Answer from the drawing. Dimensions are ordinates in mm from the lowest x, y and z of the part. Give positions to 0.01 mm unless a question says otherwise; leave off trailing zeros. Write each loop counter-clockwise with the first axis right and the second up, starting at its lowest first coordinate (ties: lowest second). Pieces come first, ordered by that corner, then holes. Notation, with made-up numbers: (50.25, -26) - (70.25, -26) arc R15 cw to (70.25, -3) - close; hole circle Ø2 at (-14.75, 9). An arc over 180 degrees is marked (long way). Write item = value, one per line.
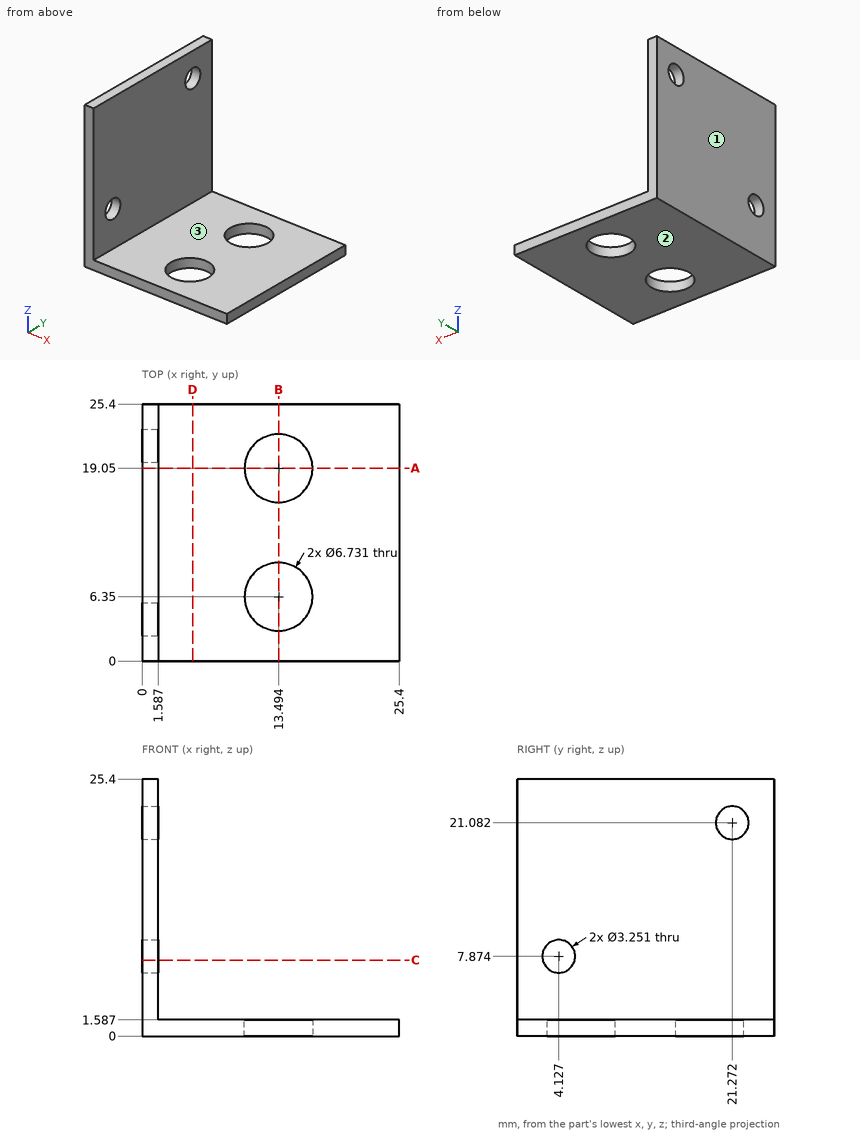
1. Find section A-A, the plane y = 19.05. Give the vertices of the cut face in (x, z).
Solution:
outline = (0, 0) - (10.13, 0) - (10.13, 1.59) - (1.59, 1.59) - (1.59, 25.4) - (0, 25.4) - close; (16.86, 0) - (25.4, 0) - (25.4, 1.59) - (16.86, 1.59) - close
2. Find section D-D, the plane x = 5. Give the vertices of the cut face in (y, z).
Solution:
outline = (0, 0) - (25.4, 0) - (25.4, 1.59) - (0, 1.59) - close
3. A straight line is drawn through the part: line 1 (Z direction, x = 11, y = 13.75). Find the intervals that lie inside material, in ascending order.
Solution:
line_1 = 0 to 1.59
4. Given pin 1 (7.5 mm diameter, centred on x = 13.49, y = 6.35, fed in from +Z); pin 2 (4 mm diameter, centred on y = 4.13, z = 7.87, fed in from +X), each flat-ended and moving along its own axis, determine where each tip first touches the part or whether it passes through.
Solution:
pin_1 = 1.59
pin_2 = 1.59
5. Find section B-B, the plane x = 13.5. Give the vertices of the cut face in (y, z) (1 decimal).
Solution:
outline = (0, 0) - (3, 0) - (3, 1.6) - (0, 1.6) - close; (9.7, 0) - (15.7, 0) - (15.7, 1.6) - (9.7, 1.6) - close; (22.4, 0) - (25.4, 0) - (25.4, 1.6) - (22.4, 1.6) - close
6. Find section C-C, the plane z = 7.5. Give the vertices of the cut face in (x, y) (1 decimal).
Solution:
outline = (0, 0) - (1.6, 0) - (1.6, 2.5) - (0, 2.5) - close; (0, 5.7) - (1.6, 5.7) - (1.6, 25.4) - (0, 25.4) - close
7. For a pull along Z with two mould halves and no side action, classify the marked faces 1, 2 and 3 as pulls with the +Z half, pulls with the -Z half, needs draft (parallel to the pull), parting line crosses it, or undercut.
Solution:
face_1 = needs draft
face_2 = pulls with the -Z half
face_3 = pulls with the +Z half
